Input: dimensioned drawing with shaded views. Units: mm. Origin: part minimum x, y, z. A direction names the side the tool comes from. Give positions to 0.01 mm unless a question says otherwise; leave off trailing zeros. Loops run counter-clockwise (first coordinate to the right, second up) from the corner with the lowest first, then second, coordinate; pieces in that order, holes last.
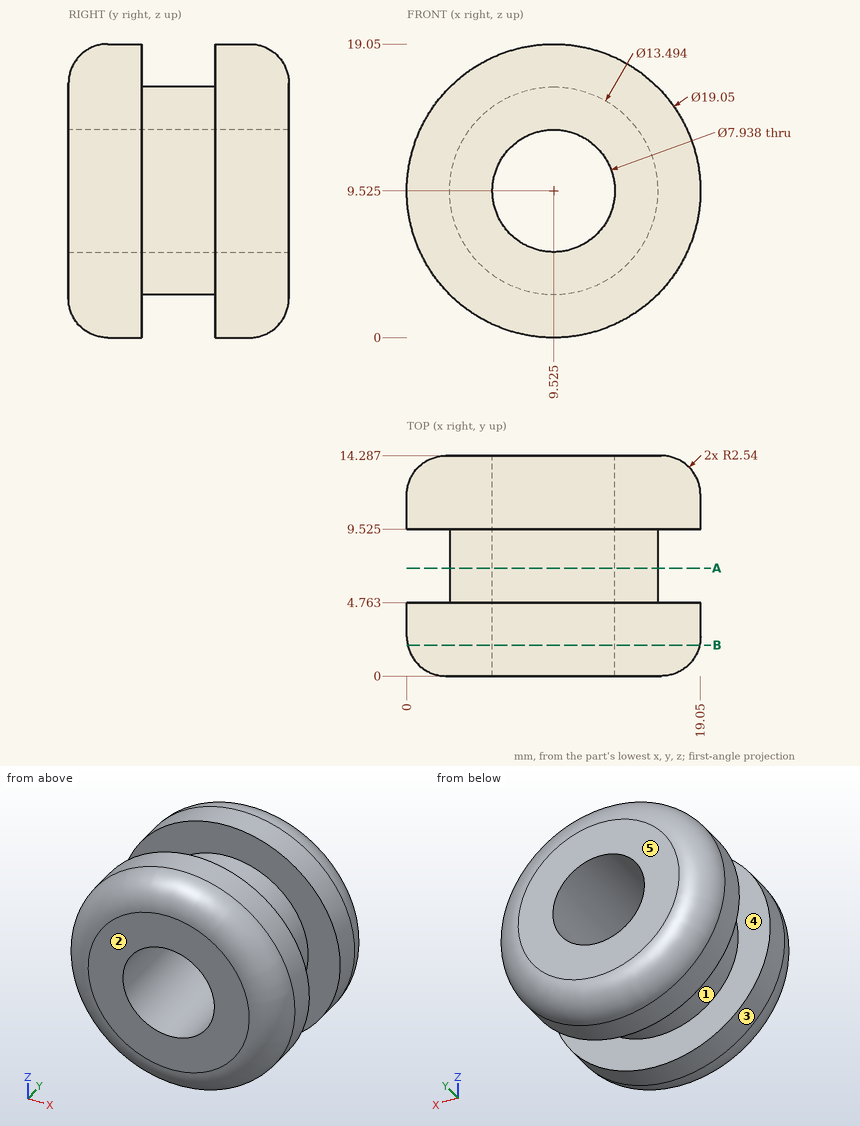
Item 1: Draft query along Y for the marked faces 1, 2 and 3. Return one class per face: +Y half, -Y half, draft (parallel to the pull), parting line (faces both ways), or undercut.
Values follow:
face 1: undercut
face 2: -Y half
face 3: draft
Item 2: Ray query, probe 1 along Y at (x, z) = (13, 2) (1 decimal); probe 2 along Z at (x, y) = (9.75, 5); probe 3 along X at (y, z) = (6.75, 4.75). Return the intervals inside material, ascending.
Values follow:
probe 1: y = 0.4 to 4.8, 9.5 to 13.9
probe 2: z = 2.78 to 5.56, 13.49 to 16.27
probe 3: x = 4.76 to 14.29
Item 3: Section query B-B on y = 2. Return loops of the section in (x, z) (1 decimal), plus the area to 3 significant figures.
Values follow:
outline: circle Ø18.9 at (9.5, 9.5); hole circle Ø7.9 at (9.5, 9.5)
area: 232 mm2
Item 4: Section query A-A on y = 7. Return loops of the section in (x, z) (1 decimal).
Values follow:
outline: circle Ø13.5 at (9.5, 9.5); hole circle Ø7.9 at (9.5, 9.5)
Item 5: Set-up query: the marked faces 4 and 5. Return all of +Z, -Z, +X, -X, +Y, -Y with unobstructed straight access to the full face (end or side cutting, diameter ignored); none if empty.
Values follow:
face 4: none
face 5: +Z, -Z, +X, -X, +Y
Item 6: Pin query (flat end, axial travel): pin 1 (1 mm diameter, centred on y = 8, z = 9, fed in from -X); pin 2 (1.5 mm diameter, centred on y = 9.5, z = 3, fed in from +X); pin 3 (4 mm diameter, centred on y = 4, z = 12.5, fed in from -X); pin 4 (7 mm diameter, centred on x = 9.525, z = 9.525, fed in from +Y). Return the tip coordinate at first contact, or that it passes through.
Values follow:
pin 1: stops at x = 2.78
pin 2: stops at x = 17.1
pin 3: stops at x = 0.05
pin 4: passes through
